Source: CAD feature listing. Evaluate the final solid. Frame: model axes, mm. Round coordinates to 2 decimals unless told otherwise and drop trailing zeros. Write each loop counter-clockwise with the first axis right and the second up, starting at its lowest first coordinate (ties: lowest second). Pieces come first, ordered by that corner, then holes. Notation, with made-up numbers: M 3.25,42 L 10.25,42 A14 cw 10.25,51 Z; hole C 77.25,44 d10. An arc over 180 degrees is marked long. Put each result on its own line as item: value. Start each with the question number.
```python
from build123d import *

# Parameters (mm, degrees)
SKETCH1_R               = 5.85
BOSS_EXTRUDE1_DEPTH     = 10
SKETCH1_4_R             = 2
CUT_EXTRUDE1_DEPTH      = 11
CUT_EXTRUDE1_DEPTH_BACK = 106


with BuildPart() as part:
    # Sketch2 → Revolve1 (revolve)
    with BuildSketch(Plane(origin=(0, 0, 0), x_dir=(0, 0, -1), z_dir=(1, 0, 0))):
        Polygon((0, -105), (7, 0), (0, 0), align=None)
    revolve(axis=Axis((0, 0, 0), (0, -1, 0)))

    # Sketch1 → Boss-Extrude1 (add)
    with BuildSketch(Plane(origin=(0, 0, 0), x_dir=(1, 0, 0), z_dir=(0, 1, 0))):
        Circle(SKETCH1_R)
    extrude(amount=BOSS_EXTRUDE1_DEPTH)

    # Sketch1<4> → Cut-Extrude1 (cut, two sides)
    with BuildSketch(Plane(origin=(0, 0, 0), x_dir=(1, 0, 0), z_dir=(0, 1, 0))) as cut_extrude1_sk:
        Circle(SKETCH1_4_R)
    extrude(amount=CUT_EXTRUDE1_DEPTH, mode=Mode.SUBTRACT)
    extrude(cut_extrude1_sk.sketch, amount=-CUT_EXTRUDE1_DEPTH_BACK, mode=Mode.SUBTRACT)


solid = part.part
```
(1) Contact query for flat-ended pins moving along their axis: P1, Ø1.5, axis at x = -2.5, y = -27, coming from the -Z side; P2, Ø4, axis at x = -3.5, y = -3, coming from the +Z side; P3, Ø1.5, axis at y = -20, z = -3, coming from the +X side. Output: stop coordinate, or through.
(2) Section query B-B (x = 0). Return loops of the section in (y, z).
(3) Section query C-C (y = -3). Return loops of the section in (x, z).
(4) Section query A-A (z = 0). Return loops of the section in (x, y).
(5) Pull-direction query (Z, two-part tool) for faces 1 (the flat face through (-6, 0, 2)), 2 (the cylindrical face through (0, -32, 2)), 3 (the cylindrical face through (-1.27, 4.93, 5.71)); classes: +Z half, -Z half, draft (parallel to the pull), parting line (faces both ways), or undercut.
(6) Section query D-D (y = -31.5). Return loops of the section in (x, z).
(7) Ray query, line 1 along Z through (x, y) = (0, -55); line 2 along X through (y, z) = (-4.5, -0.75); line 3 along X through (y, z) = (-23.5, 0.75). Return the intervals inside material, ascending.
Entries:
1. P1: z = -4.9
1. P2: z = 6.65
1. P3: x = 5.21
2. outline: M -75,-2 L 0,-7 L 0,-5.85 L 10,-5.85 L 10,-2 Z; M -75,2 L 10,2 L 10,5.85 L 0,5.85 L 0,7 Z
3. outline: C 0,0 d13.6; hole C 0,0 d4
4. outline: M -7,0 L -2,-75 L -2,10 L -5.85,10 L -5.85,0 Z; M 2,-75 L 7,0 L 5.85,0 L 5.85,10 L 2,10 Z
5. face 1: draft
5. face 2: undercut
5. face 3: parting line
6. outline: C 0,0 d9.8; hole C 0,0 d4
7. line 1: -3.33 to -2, 2 to 3.33
7. line 2: -6.66 to -1.85, 1.85 to 6.66
7. line 3: -5.38 to -1.85, 1.85 to 5.38
